from build123d import *

# Parameters (mm, degrees)
SKETCH_1_W          = 10
SKETCH_1_H          = 10
SKETCH_1_W_2        = 6.4
SKETCH_1_H_2        = 7
EXTRUDE_1_DEPTH     = 63
SKETCH_2_R          = 1.5
CUT_EXTRUDE_1_DEPTH = 30
SKETCH_3_R          = 2
CUT_EXTRUDE_2_DEPTH = 30


with BuildPart() as part:
    # 草图1 → 凸台-拉伸1 (new body)
    with BuildSketch(Plane(origin=(0, 0, 0), x_dir=(1, 0, 0), z_dir=(0, 1, 0))):
        Rectangle(SKETCH_1_W, SKETCH_1_H)
        Rectangle(SKETCH_1_W_2, SKETCH_1_H_2, mode=Mode.SUBTRACT)
    extrude(amount=EXTRUDE_1_DEPTH)

    # 草图2 → 切除-拉伸1 (cut)
    with BuildSketch(Plane.XY.offset(5)):
        with Locations((0, 41.5)):
            Circle(SKETCH_2_R)
        with Locations((0, 21.5)):
            Circle(SKETCH_2_R)
    extrude(amount=-CUT_EXTRUDE_1_DEPTH, mode=Mode.SUBTRACT)

    # 草图3 → 切除-拉伸2 (cut)
    with BuildSketch(Plane(origin=(5, 0, 0), x_dir=(0, 0, -1), z_dir=(1, 0, 0))):
        with Locations((0, 5)):
            Circle(SKETCH_3_R)
        with Locations((0, 58)):
            Circle(SKETCH_3_R)
    extrude(amount=-CUT_EXTRUDE_2_DEPTH, mode=Mode.SUBTRACT)


solid = part.part
The listing builds one solid part. Answer for the finished solid, in the listing's coordinates (mm). A direction names the side the tool comes from. Give positions to 0.01 mm unless a question says otherwise; leave off trailing zeros. Order: outer loops, then holes, each group sorted by start corner. A loop starts at its lowest first (then second) coordinate and runs counter-clockwise, first axis right, second up. Notation, with made-up numbers: (32, 28.25) - (39, 28.25) arc R16 cw to (39, 54.25) - close; hole circle Ø4 at (-19.5, -34). An arc over 180 degrees is marked (long way). Answer as CSV lines item,"result".
Q1. A cutting plane is placed at A-A, the plane x = 0. Determine the outline of the cut face in (y, z), and give its area (3 significant figures).
Answer key:
outline,"(0, -5) - (20, -5) - (20, -3.5) - (0, -3.5) - close; (0, 3.5) - (20, 3.5) - (20, 5) - (0, 5) - close; (23, -5) - (40, -5) - (40, -3.5) - (23, -3.5) - close; (23, 3.5) - (40, 3.5) - (40, 5) - (23, 5) - close; (43, -5) - (63, -5) - (63, -3.5) - (43, -3.5) - close; (43, 3.5) - (63, 3.5) - (63, 5) - (43, 5) - close"
area,"171 mm^2"
Q2. A cutting plane is placed at D-D, the plane y = 51. Determine the outline of the cut face in (x, z), and give its area (3 significant figures).
Answer key:
outline,"(-5, -5) - (5, -5) - (5, 5) - (-5, 5) - close; hole (-3.2, -3.5) - (3.2, -3.5) - (3.2, 3.5) - (-3.2, 3.5) - close"
area,"55.2 mm^2"
Q3. Straight lines are drawn through the part: L1, parallel to Y at x = 0, z = 4.75; L2, parallel to Y at x = 3.75, z = 0; L3, parallel to X at y = 34, z = -1.25. For each, find the intervals that lie inside material, in ascending order.
Answer key:
L1,"y = 0 to 20, 23 to 40, 43 to 63"
L2,"y = 0 to 3, 7 to 56, 60 to 63"
L3,"x = -5 to -3.2, 3.2 to 5"
Q4. This flat-tipped pin is pushed along its axis until it touches: pin 1 Ø3 at (y, z) = (58, 0) entering from +X. Where does it stop, or does it pass through?
Answer key:
pin 1,"passes through"
Q5. A cutting plane is placed at B-B, the plane y = 21.5. Determine the outline of the cut face in (x, z).
Answer key:
outline,"(-5, -5) - (-1.5, -5) - (-1.5, -3.5) - (-3.2, -3.5) - (-3.2, 3.5) - (-1.5, 3.5) - (-1.5, 5) - (-5, 5) - close; (1.5, -5) - (5, -5) - (5, 5) - (1.5, 5) - (1.5, 3.5) - (3.2, 3.5) - (3.2, -3.5) - (1.5, -3.5) - close"
Q6. Determine the mould class of faces 1 (the face through (4, 7, 0)), 2 (the face through (5, 31, 0)), 3 (the face through (0, 40, -4)), 4 (the face through (-5, 31, 0)) for opening direction X: pulls with the +X half, pulls with the -X half, needs draft (parallel to the pull), parting line crosses it, or undercut.
Answer key:
face 1,"needs draft"
face 2,"pulls with the +X half"
face 3,"undercut"
face 4,"pulls with the -X half"
Q7. Which of the six approach directions +Z, -Z, +X, -X, +Y, -Y give full straight-line access (tool end or side, diameter ignored) to faces 5 (the face through (-3.4, 0, -0.1)), 6 (the face through (-3.2, 31, 0))?
Answer key:
face 5,"+Z, -Z, +X, -X, -Y"
face 6,"+Y, -Y"
Q8. A cutting plane is placed at C-C, the plane z = 1. Determine the outline of the cut face in (x, y), and give its area (3 significant figures).
Answer key:
outline,"(-5, 0) - (-3.2, 0) - (-3.2, 3.27) - (-5, 3.27) - close; (-5, 6.73) - (-3.2, 6.73) - (-3.2, 56.27) - (-5, 56.27) - close; (-5, 59.73) - (-3.2, 59.73) - (-3.2, 63) - (-5, 63) - close; (3.2, 0) - (5, 0) - (5, 3.27) - (3.2, 3.27) - close; (3.2, 6.73) - (5, 6.73) - (5, 56.27) - (3.2, 56.27) - close; (3.2, 59.73) - (5, 59.73) - (5, 63) - (3.2, 63) - close"
area,"202 mm^2"
